Could you check a few things on this model? Use its own coordinates, in mm. Face numbers are marked on the shaded views. A direction names the side the tool comes from. Give positions to 0.01 mm unless a question says otherwise; leave off trailing zeros. Order: outer loops, then holes, each group sorted by start corner. A loop starts at its lowest first (then second) coordinate and runs counter-clockwise, first axis right, second up. Notation, with made-up numbers: (14, 40) - (23, 40) arc R11 ccw to (23, 48) - close; hole circle Ø6 at (89, -5.5). An arc over 180 degrees is marked (long way). Put each result on its own line as item: value.
from build123d import *

# Parameters (mm, degrees)
F0_W     = 38.1
F0_H     = 6.35
F1_DEPTH = 25.4
F2_W     = 25.4
F2_H     = 6.35
F3_DEPTH = 12.7
F4_R     = 12.7
F5_DEPTH = 12.7


with BuildPart() as f1:
    # F0 (on Front) → F1 (new body)
    with BuildSketch(Plane.XZ):
        with Locations((19.05, 3.175)):
            Rectangle(F0_W, F0_H)
    extrude(amount=F1_DEPTH)

    # F2 (on Right) → F3 (join)
    with BuildSketch(Plane.YZ):
        with Locations((-12.7, 9.525)):
            Rectangle(F2_W, F2_H)
    extrude(amount=F3_DEPTH)

    # F4 (on Right) → F5 (join)
    with BuildSketch(Plane.YZ):
        with Locations((-12.706821, 12.748167)):
            Circle(F4_R)
    extrude(amount=F5_DEPTH)


solid = f1.part
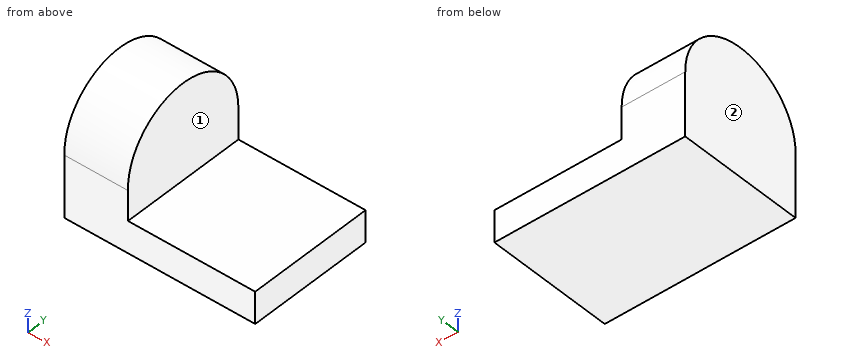
1) I'm going to push flat-ended pins straight in: pin 1 (10 mm diameter, centred on y = -8, z = 18.5, fed in from +X); pin 2 (12 mm diameter, centred on x = 6.5, z = 22.5, fed in from -Y); pin 3 (1 mm diameter, centred on x = 25.5, y = -21.5, fed in from +Z). Where does each tip first touch, or does it pass through?
Filled in:
pin 1: stops at x = 12.7
pin 2: stops at y = -24.84
pin 3: stops at z = 6.35
2) Suppose I cut it at B-B, the plane y = -21. List the corners of the cut face in (x, z) for me.
Filled in:
outline: (0, 0) - (38.1, 0) - (38.1, 6.35) - (12.7, 6.35) - (12.7, 22.37) - (0, 22.37) - close
3) If I drill on line 1 (Z direction, x = 23.5, y = -4.5); line 2 (X direction, y = -4, z = 21.5); line 3 (Y direction, x = 10, z = 6.5), over which ranges is the centre line in solid material (lowest first)? Write a range as [from, to].
Filled in:
line 1: z = [0, 6.35]
line 2: x = [0, 12.7]
line 3: y = [-25.4, 0]
4) Suppose I cut it at D-D, the plane y = -3.25. List the corners of the cut face in (x, z) for me.
Filled in:
outline: (0, 0) - (38.1, 0) - (38.1, 6.35) - (12.7, 6.35) - (12.7, 21.23) - (0, 21.23) - close
5) Suppose I cut it at C-C, the plane z = 21. List the corners of the cut face in (x, y) for me, and give its area (3 significant figures).
Filled in:
outline: (0, -22.36) - (12.7, -22.36) - (12.7, -3.05) - (0, -3.05) - close
area: 245 mm^2
6) Which directions (+Z, -Z, +X, -X, +Y, -Y) give clear straight access to the entire face, cutting with the end or side of a thin tool? Please do the marked faces 1 and 2.
Filled in:
face 1: +Z, +X, +Y, -Y
face 2: +Z, -Z, -X, +Y, -Y
